Here's how the part is built. I have some questions about the finished solid (model axes, mm). Face numbers are marked on the shaded views. Round coordinates to 2 decimals unless told otherwise and drop trailing zeros. Write each loop counter-clockwise with the first axis right and the second up, starting at its lowest first coordinate (ties: lowest second). Pieces come first, ordered by that corner, then holes. Notation, with made-up numbers: (10, -17.75) - (55, -17.75) arc R21 cw to (55, 3.25) - close; hole circle Ø11 at (-8, 83). An arc over 180 degrees is marked (long way). One line per item, written item: value. Start each with the question number.
Item 1: For P1, Ø4, axis at x = -2, z = 7, coming from the +Y side; P2, Ø2, axis at y = 34.5, z = 22.5, coming from the +X side; P3, Ø2, axis at x = -21, z = 25.5, coming from the +Y side, each with a flat end and sliding along its axis, tell me the tip position at first contact or that it passes through.
Item 2: If I drill on line 1 (X direction, y = 8.5, z = 9.5); line 2 (Y direction, x = -2.5, z = 5.5); line 3 (Z direction, x = 16, y = 7), over which ranges is the centre line in solid material (lowest first)?
Item 3: Imagine slicing it at B-B, the plane z = 12. Please give me the cut outline in (x, y).
Item 4: Imagine slicing it at A-A, the plane z = 6. Please give me the cut outline in (x, y).
Item 5: Thinking about a two-plate mould opening in X: for the marked faces 1, 2 and 3, which applies, released by +X, released by -X, zero draft, split by the parting line, or undercut?
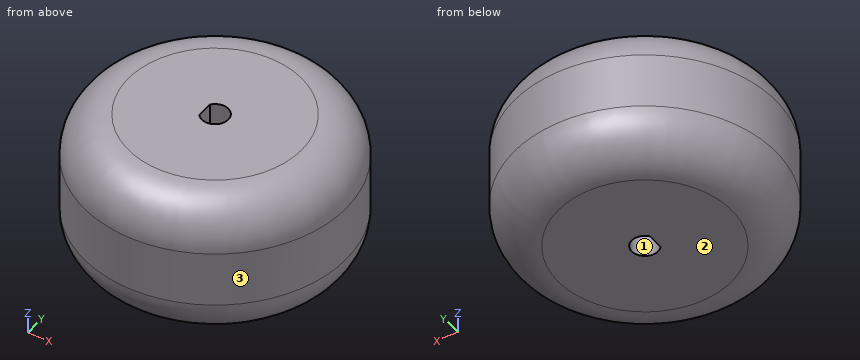
```python
from build123d import *

# Parameters (mm, degrees)
ESQUISSE1_R             = 29.65
BOSS_EXTRU_1_DEPTH      = 32.63
ESQUISSE3_R             = 3
ENL_V_MAT_EXTRU_1_DEPTH = 33.63
ESQUISSE4_W             = 2.697553301
ESQUISSE4_H             = 5.967314877
BOSS_EXTRU_4_DEPTH      = 32.63
CONG_1_R                = 10
CONG_2_R                = 10


with BuildPart() as part:
    # Esquisse1 → Boss.-Extru.1 (new body)
    with BuildSketch(Plane.XY):
        with Locations((-8.87201182, 11.161610959)):
            Circle(ESQUISSE1_R)
    extrude(amount=BOSS_EXTRU_1_DEPTH)

    # Esquisse3 → Enlèv. mat.-Extru.1 (cut)
    with BuildSketch(Plane.XY.offset(32.63)):
        with Locations((-8.87201182, 11.161610959)):
            Circle(ESQUISSE3_R)
    extrude(amount=-ENL_V_MAT_EXTRU_1_DEPTH, mode=Mode.SUBTRACT)

    # Esquisse4 → Boss.-Extru.4 (add)
    with BuildSketch(Plane.XY.offset(32.63)):
        with Locations((-12.590788471, 11.037032126)):
            Rectangle(ESQUISSE4_W, ESQUISSE4_H)
    extrude(amount=-BOSS_EXTRU_4_DEPTH)

    # Congé1
    cong_1_edges = [part.edges().sort_by_distance(p)[0] for p in [
        (-38.52201182, 11.161610959, 0),
    ]]
    fillet(cong_1_edges, radius=CONG_1_R)

    # Congé2
    cong_2_edges = [part.edges().sort_by_distance(p)[0] for p in [
        (-38.52201182, 11.161610959, 32.63),
    ]]
    fillet(cong_2_edges, radius=CONG_2_R)


solid = part.part
```
Values follow:
1. P1: stops at y = 40.18
1. P2: stops at x = 10.62
1. P3: stops at y = 38.28
2. line 1: x = -38.39 to -10.26, -7.49 to 20.65
2. line 2: y = -16.7 to 39.02
2. line 3: z = 1.69 to 30.94
3. outline: circle Ø59.3 at (-8.87, 11.16); hole (-11.24, 9.32) arc R3 ccw (long way) to (-11.24, 13) - close
4. outline: circle Ø57.63 at (-8.87, 11.16); hole (-11.24, 9.32) arc R3 ccw (long way) to (-11.24, 13) - close
5. face 1: undercut
5. face 2: zero draft
5. face 3: split by the parting line
